Build history of the part. All positions in model axes, mm. Coordinates: 2 decimals unless noted, no trailing zeros. Loops run counter-clockwise (first coordinate to the right, second up) from the corner with the lowest first, then second, coordinate; pieces in that order, holes last.
Item 1: Drill centre lines: line 1 along Z through (x, y) = (1, 3); line 2 along Y through (x, z) = (1.9, -70); line 3 along Y through (x, z) = (0.85, -46.5). Where is each one in solid material? Low to high.
Item 2: Cut at D-D (z = -2). List the corners of the cut face in (x, y), and give its area (3 significant figures).
Item 3: Flat gauge pin, fed straight in: pin 1 (6 mm diameter, centred on y = 5, z = -51.5, fed in from -X). Where does the tip first touch, or does it go through?
Item 4: Cut at A-A (y = 6.5). List the corners of the cut face in (x, z).
Item 5: Cut at C-C (x = 1.7). List the corners of the cut face in (y, z) (3 decimals), and give its area (3 significant figures).
Item 6: Cut at B-B (z = -13.5). List the corners of the cut face in (x, y).
from build123d import *

# Parameters (mm, degrees)
SKETCH_1_R      = 0.5
EXTRUDE_1_DEPTH = 2
SKETCH_2_R      = 0.5
EXTRUDE_2_DEPTH = 2


with BuildPart() as part:
    # 草图1 → 凸台-拉伸1 (new body)
    with BuildSketch(Plane(origin=(0, 0, 0), x_dir=(0, 0, -1), z_dir=(1, 0, 0))):
        with BuildLine():
            Line((-8.746696486, 4.522861275), (75.253303514, 4.522861275))
            ThreePointArc((75.253303514, 4.522861275), (76.753303514, 3.022861275), (75.253303514, 1.522861275))
            Line((75.253303514, 1.522861275), (-8.746696486, 1.522861275))
            ThreePointArc((-8.746696486, 1.522861275), (-10.246696486, 3.022861275), (-8.746696486, 4.522861275))
        make_face()
        with Locations((-8.746696486, 3.022861275)):
            Circle(SKETCH_1_R, mode=Mode.SUBTRACT)
        with Locations((75.253303514, 3.022861275)):
            Circle(SKETCH_1_R, mode=Mode.SUBTRACT)
    extrude(amount=EXTRUDE_1_DEPTH)

    # 草图2 → 凸台-拉伸2 (add)
    with BuildSketch(Plane.ZY):
        with BuildLine():
            Line((-62.171828062, 18.22565707), (-76.313963686, 4.083521447))
            ThreePointArc((-76.313963686, 4.083521447), (-76.313963686, 1.962201103), (-74.192643342, 1.962201103))
            Line((-74.192643342, 1.962201103), (-60.619757708, 15.535086737))
            Line((-60.619757708, 15.535086737), (8.449071616, 1.552684606))
            ThreePointArc((8.449071616, 1.552684606), (10.216873155, 2.725236404), (9.044321357, 4.493037943))
            Line((9.044321357, 4.493037943), (-60.81354302, 18.635173567))
            ThreePointArc((-60.81354302, 18.635173567), (-61.544159412, 18.601143946), (-62.171828062, 18.22565707))
        make_face()
        with Locations((-61.11116789, 17.164996899)):
            Circle(SKETCH_2_R, mode=Mode.SUBTRACT)
        with Locations(Location((-75.253303514, 3.022861275, 0), (0, 0, 180))):
            Circle(SKETCH_2_R, mode=Mode.SUBTRACT)
        with Locations(Location((8.746696486, 3.022861275, 0), (0, 0, 180))):
            Circle(SKETCH_2_R, mode=Mode.SUBTRACT)
    extrude(amount=-EXTRUDE_2_DEPTH)


solid = part.part
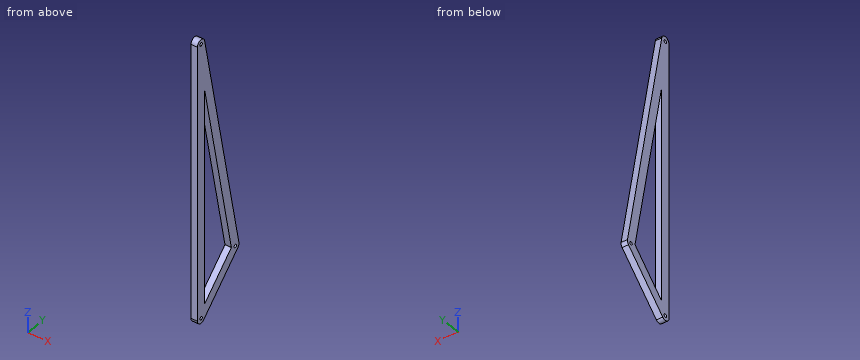
Filled sheet:
1. line 1: z = -76.75 to -75.75, -74.75 to 8.25, 9.25 to 10.25
1. line 2: y = 1.52 to 4.52, 6.15 to 10.4
1. line 3: y = 1.52 to 4.52, 12.68 to 15.74
2. outline: (0, 1.52) - (2, 1.52) - (2, 6.73) - (0, 6.73) - close
2. area: 10.4 mm2
3. pin 1: stops at x = 0
4. outline: (0, -73.9) - (2, -73.9) - (2, -69.65) - (0, -69.65) - close; (0, -15.99) - (2, -15.99) - (2, -0.87) - (0, -0.87) - close
5. outline: (1.523, -75.253) arc R1.5 ccw to (4.084, -76.314) - (18.226, -62.172) arc R1.5 ccw to (18.635, -60.814) - (4.493, 9.044) arc R1.5 ccw to (1.523, 8.747) - close; hole circle Ø1 at (3.023, -75.253); hole circle Ø1 at (3.023, 8.747); hole (4.523, -71.632) - (15.535, -60.62) - (4.523, -6.223) - close; hole circle Ø1 at (17.165, -61.111)
5. area: 501 mm2
6. outline: (0, 1.52) - (2, 1.52) - (2, 4.52) - (0, 4.52) - close; (0, 6) - (2, 6) - (2, 9.06) - (0, 9.06) - close
